```python
from build123d import *

# Parameters (mm, degrees)
SKETCH011_R       = 2.5
PAD009_DEPTH      = 5.6
CYLINDER006_R     = 4
CYLINDER006_DEPTH = 8
CYLINDER007_R     = 5
CYLINDER007_DEPTH = 10


with BuildPart() as part:
    # Sketch011 → Pad009 (new body)
    with BuildSketch(Plane.XZ.offset(3.2)):
        with BuildLine():
            ThreePointArc((-0.801584, 57.426821), (3.495987, 60.666233), (-0.47207, 64.301812))
            Line((-9.631324, 59.476576), (-0.47207, 64.301812))
            ThreePointArc((-9.631324, 59.476576), (-10.211746, 53.667403), (-4.638391, 55.405532))
            Line((-4.638391, 55.405532), (-0.801584, 57.426821))
        make_face()
        with Locations((-8, 56.38)):
            Circle(SKETCH011_R, mode=Mode.SUBTRACT)
        with Locations((0, 60.833794)):
            Circle(SKETCH011_R, mode=Mode.SUBTRACT)
    extrude(amount=PAD009_DEPTH)

    # Cylinder006 → Cylinder006 (cut)
    with BuildSketch(Plane(origin=(-8, 1.8, 56), x_dir=(1, 0, 0), z_dir=(0, -1, 0))):
        Circle(CYLINDER006_R)
    extrude(amount=CYLINDER006_DEPTH, mode=Mode.SUBTRACT)

    # Cylinder007 → Cylinder007 (cut)
    with BuildSketch(Plane(origin=(0, -7.4, 61), x_dir=(1, 0, 0), z_dir=(0, -1, 0))):
        Circle(CYLINDER007_R)
    extrude(amount=CYLINDER007_DEPTH, mode=Mode.SUBTRACT)


solid = part.part
```
Geometry check sheet. Reference: the model listing, model coordinates, mm. A direction names the side the tool comes from. Coordinates: 2 decimals unless noted, no trailing zeros. Loops run counter-clockwise (first coordinate to the right, second up) from the corner with the lowest first, then second, coordinate; pieces in that order, holes last. Notation, with made-up numbers: (32.25, -16) -> (61.25, -16) arc R22 ccw to (61.25, 7) -> close; hole circle Ø2 at (-10.5, 69.5). An arc over 180 degrees is marked (long way). Put each result on its own line as item: value.
1) Gauge pin test, flat ends, axial feed: pin 1 Ø6.5 at (x, z) = (-8, 56.38) entering from +Y; pin 2 Ø4 at (x, z) = (-0.5, 62) entering from -Y; pin 3 Ø2 at (x, y) = (0.5, -4.5) entering from -Z. Record the tip position at first contact, or that the pin passes through.
Result set:
pin 1: stops at y = -6.2
pin 2: stops at y = -7.4
pin 3: stops at z = 57.33
2) Tool access check on faces 1 (the flat face through (-5.116, -5.961, 61.855)), 2 (the cylindrical face through (-4.541, -8.09, 58.906)). Record the directions out of +Z, -Z, +X, -X, +Y, -Y that give a thin tool (end or side, any length) a straight path to the whole face; none if there is none.
Result set:
face 1: +Z, -X, +Y, -Y
face 2: +X, -Y
3) Thickness scan on line 1 (Z direction, x = 0, y = -5.05); line 2 (Y direction, x = -7, z = 59.5); line 3 (X direction, y = -4.2, z = 59). Record the ranges inside material, lowest first.
Result set:
line 1: z = 57.33 to 58.33, 63.33 to 64.33
line 2: y = -8.8 to -6.2
line 3: x = -5.35 to -1.7, 1.7 to 2.98
4) Cross-section at B-B on z = 56.38. Record the boundary of the cut face in (x, y), plus the area to 3 significant figures.
Result set:
outline: (-11.5, -8.8) -> (-10.5, -8.8) -> (-10.5, -6.2) -> (-11.5, -6.2) -> close; (-5.5, -8.8) -> (-2.79, -8.8) -> (-2.79, -3.2) -> (-4.02, -3.2) -> (-4.02, -6.2) -> (-5.5, -6.2) -> close
area: 13.3 mm^2
5) Release check for a two-part mould opening along X. For faces 3 (the flat face through (-3, -7.4, 61)), 4 (the cylindrical face through (-9.84, -7.48, 58.07)), 5 (the cylindrical face through (-10.286, -7.482, 53.73)) record: released by +X, released by -X, zero draft, split by the parting line, or undercut.
Result set:
face 3: zero draft
face 4: undercut
face 5: split by the parting line
6) Cross-section at C-C on y = -6.5. Record the boundary of the cut face in (x, z).
Result set:
outline: (-9.63, 59.48) arc R3.5 ccw (long way) to (-4.64, 55.41) -> (-0.8, 57.43) arc R3.5 ccw (long way) to (-0.47, 64.3) -> close; hole circle Ø5 at (-8, 56.38); hole circle Ø5 at (0, 60.83)
7) Cross-section at D-D on x = -6. Record the boundary of the cut face in (y, z).
Result set:
outline: (-8.8, 53.51) -> (-6.2, 53.51) -> (-6.2, 54.88) -> (-8.8, 54.88) -> close; (-8.8, 57.88) -> (-6.2, 57.88) -> (-6.2, 59.46) -> (-3.2, 59.46) -> (-3.2, 61.39) -> (-8.8, 61.39) -> close
8) Cross-section at A-A on x = 0. Record the boundary of the cut face in (y, z).
Result set:
outline: (-7.4, 57.33) -> (-3.2, 57.33) -> (-3.2, 58.33) -> (-7.4, 58.33) -> close; (-7.4, 63.33) -> (-3.2, 63.33) -> (-3.2, 64.33) -> (-7.4, 64.33) -> close
